Can you work these out from the model? Positions are in its coordinate system, mm. A direction names the side the tool comes from. Give positions to 0.01 mm unless a question says otherwise; leave off trailing zeros. Order: outer loops, then holes, each group sorted by start corner. A loop starts at its lowest first (then second) coordinate and runs counter-clockwise, first axis right, second up. Notation, with made-up numbers: (76.5, -28) - (91.5, -28) arc R35 cw to (91.5, 9) - close; hole circle Ø2 at (-12.5, 80.5). An arc over 180 degrees is marked (long way). Return JSON: item names as keys, results as strings.
```python
from build123d import *

# Parameters (mm, degrees)
CHAMFER1_SIZE           = 0.8
CUT_EXTRUDE1_DEPTH      = 6
CUT_EXTRUDE2_DEPTH      = 21
CUT_EXTRUDE2_DEPTH_BACK = 18
SKETCH17_W              = 9.291812213
SKETCH17_H              = 14.847741165
CUT_EXTRUDE3_DEPTH      = 18
CUT_EXTRUDE3_DEPTH_BACK = 18
SKETCH18_W              = 16.942014586
SKETCH18_H              = 5.743756165
CUT_EXTRUDE4_DEPTH      = 36
CUT_EXTRUDE4_DEPTH_BACK = 60
SKETCH19_W              = 5.251267682
SKETCH19_H              = 11.080799959


with BuildPart() as part:
    # Sketch1 → Revolve1 (revolve)
    with BuildSketch(Plane(origin=(0, 0, 0), x_dir=(0, 0, -1), z_dir=(1, 0, 0)), mode=Mode.PRIVATE) as revolve1_sk:
        Polygon((0, 0), (0, 5.618156666), (0.538, 6.55), (7.462, 6.55), (8, 5.618156666), (8, 4), (38, 4), (38, 0), align=None)
    revolve(revolve1_sk.sketch.rotate(Axis((0, 0, 0), (0, 0, -1)), 90), axis=Axis((0, 0, 0), (0, 0, -1)))

    # Chamfer1
    chamfer1_edges = [part.edges().sort_by_distance(p)[0] for p in [
        (-4, 0, -38),
    ]]
    chamfer(chamfer1_edges, length=CHAMFER1_SIZE)

    # Sketch2 → Cut-Extrude1 (cut)
    with BuildSketch(Plane.XY):
        Polygon((3.25, 1.876388375), (0, 3.75277675), (-3.25, 1.876388375), (-3.25, -1.876388375), (0, -3.75277675), (3.25, -1.876388375), align=None)
    extrude(amount=-CUT_EXTRUDE1_DEPTH, mode=Mode.SUBTRACT)

    # Sketch3 → Cut-Revolve1 (revolve, cut)
    with BuildSketch(Plane(origin=(0, 0, 0), x_dir=(0, 0, -1), z_dir=(1, 0, 0)), mode=Mode.PRIVATE) as cut_revolve1_sk:
        Polygon((0, 0), (0, 4), (2.309401077, 0), align=None)
        Polygon((6, 0), (6, 3.75277675), (8.166666667, 0), align=None)
    revolve(cut_revolve1_sk.sketch.rotate(Axis((0, 0, 1.402800488), (0, 0, -1)), 90), axis=Axis((0, 0, 1.402800488), (0, 0, -1)), mode=Mode.SUBTRACT)

    # Sketch17 → Cut-Extrude2 (cut, two sides: drawn at the far end of the back side and taken through both)
    with BuildSketch(Plane.ZY.offset(-3.25).offset(-CUT_EXTRUDE2_DEPTH_BACK)):
        with Locations((-34.32554678, -0.925988159)):
            Rectangle(SKETCH17_W, SKETCH17_H)
    extrude(amount=CUT_EXTRUDE2_DEPTH + CUT_EXTRUDE2_DEPTH_BACK, mode=Mode.SUBTRACT)

    # Sketch18 → Cut-Extrude3 (cut, two sides: drawn at the far end of the back side and taken through both)
    with BuildSketch(Plane(origin=(1.625, 2.814582562, 0), x_dir=(0.8660254037844387, -0.49999999999999983, 0), z_dir=(-0.49999999999999983, -0.8660254037844387, 0)).offset(-CUT_EXTRUDE3_DEPTH_BACK)):
        with Locations((1.337252905, -27.251034813)):
            Rectangle(SKETCH18_W, SKETCH18_H)
    extrude(amount=CUT_EXTRUDE3_DEPTH + CUT_EXTRUDE3_DEPTH_BACK, mode=Mode.SUBTRACT)

    # Sketch19 → Cut-Extrude4 (cut, two sides: drawn at the far end of the back side and taken through both)
    with BuildSketch(Plane(origin=(0, 0, 0), x_dir=(0, 0, -1), z_dir=(1, 0, 0)).offset(-CUT_EXTRUDE4_DEPTH_BACK)):
        with Locations((21.973190176, -0.187545275)):
            Rectangle(SKETCH19_W, SKETCH19_H)
    extrude(amount=CUT_EXTRUDE4_DEPTH + CUT_EXTRUDE4_DEPTH_BACK, mode=Mode.SUBTRACT)


solid = part.part
```
1. On a 3-axis mill with a long thin cutter (end or side, diameter ignored), from which of +Z, -Z, +X, -X, +Y, -Y can I reach the whole of each face in a straight line? I mean faces 1 (the face through (-1.7, -3, -6)), 2 (the face through (2, 4, -8)), 3 (the face through (1.6, -2.83, -3.03)). Say none if no direction works.
Checks:
{"face 1": "none", "face 2": "-Z", "face 3": "+Z"}
2. Suppose I cut it at B-B (z = -10.75). List the corners of the cut face in (x, y) for me.
Checks:
{"outline": "circle Ø8 at (0, 0)"}
3. Thinking about a two-plate mould opening in Y: for faces 4 (the face through (-4.828, -4.427, -4.048)), 5 (the face through (0, 0, -19.348)), 6 (the face through (1.65, 2.8, -3.03)), which applies, +Y half, -Y half, draft (parallel to the pull), parting line (faces both ways), or undercut?
Checks:
{"face 4": "parting line", "face 5": "draft", "face 6": "undercut"}
4. For pin 1 Ø1.9 at (y, z) = (1, -2.5) entering from +X; pin 2 Ø6 at (x, z) = (2, -10) entering from +Y; pin 3 Ø6 at (x, z) = (5, -9) entering from +Y; pin 4 Ø5 at (y, z) = (2, -11) entering from +X, each with a flat end and sliding along its axis, tell me the tip position at first contact or that it passes through.
Checks:
{"pin 1": "x = 6.55", "pin 2": "y = 6.54", "pin 3": "y = 6.08", "pin 4": "x = 4"}
5. If I drill on L1, parallel to Z at x = 2, y = 4.75; L2, parallel to X at y = 2.5, z = -2.5; L3, parallel to Y at x = 1.75, z = -5.25, over which ranges is the centre line in solid material (lowest first)? Write a range as [from, to].
Checks:
{"L1": "[-8, 0]", "L2": "[-6.05, -2.17], [2.17, 6.05]", "L3": "[-6.31, -2.74], [2.74, 6.31]"}
6. Suppose I cut it at A-A (z = -4). List the corners of the cut face in (x, y) for me, plus the area to 3 significant figures.
Checks:
{"outline": "circle Ø13.1 at (0, 0); hole (-3.25, -1.88) - (0, -3.75) - (3.25, -1.88) - (3.25, 1.88) - (0, 3.75) - (-3.25, 1.88) - close", "area": "98.2 mm^2"}
